Input: part model. Units: mm. Frame: model coordinates. A direction names the side the tool comes from. Round coordinates to 2 decimals unless told otherwise and drop trailing zeros. Loops run counter-clockwise (first coordinate to the right, second up) from the corner with the lowest first, then second, coordinate; pieces in that order, holes last.
1) Ray query, line 1 along X through (y, z) = (82, 29.5); line 2 along X through (y, z) = (100, 28); line 3 along Z through (x, y) = (10.5, 105.5). Return the intervals inside material, ascending.
2) Draft query along X for faces 3 (the face through (1.87, 75.13, 88.88)), 4 (the face through (0.1, 75.1, 76.2)), 5 (the face through (0, 152.4, 78)). Return one class per face: pulls with the +X half, pulls with the -X half, needs draft (parallel to the pull), parting line crosses it, or undercut.
3) Section B-B, the plane z = 65. Return loops of the section in (x, y), and give its area (3 significant figures).
4) Access query for faces 1 (the face through (0, 0, 78)), 2 (the face through (58.95, 75.13, 57.79)). Directions: +Z, -Z, +X, -X, +Y, -Y. A direction counts if a zero-diameter tool reaches every point of the face in a straight line with its end or side. Return the directions, or none.
5) First-contact query: pin 1 (1.5 mm diameter, centred on y = 99, z = 43, fed in from +X); pin 2 (0.6 mm diameter, centred on x = 82.5, y = 42.5, fed in from -Z); pin 3 (0.6 mm diameter, centred on x = -88.5, y = 108.5, fed in from -Z). Flat tips, straight axial feed; report the tip coordinate or a pass-through.
6) Section A-A, the plane y = 99.5. Return loops of the section in (x, z).
7) Section C-C, the plane z = 38. Return loops of the section in (x, y).
8) Section D-D, the plane x = -49.5. Return loops of the section in (y, z).
from build123d import *

# Parameters (mm, degrees)
F0_R     = 88.9
F1_DEPTH = 152.4
F4_DEPTH = 152.401
F5_DEPTH = 152.401
F7_DEPTH = 152.401


with BuildPart() as f1:
    # F0 (on Front) → F1 (new body)
    with BuildSketch(Plane.XZ):
        Circle(F0_R)
    extrude(amount=-F1_DEPTH)

    # F3 (on face) → F4 (cut, through all)
    with BuildSketch(Plane.XZ):
        with BuildLine():
            ThreePointArc((6.3453015162, 82.3057692308), (0, 76.2), (-6.3453015162, 82.3057692308))
            ThreePointArc((-6.3453015162, 82.3057692308), (-58.3716647869, 58.3716647869), (-82.3057692308, 6.3453015162))
            ThreePointArc((-82.3057692308, 6.3453015162), (-77.974338005, 4.4029328075), (-76.2, 0))
            ThreePointArc((-76.2, 0), (-77.974338005, -4.4029328075), (-82.3057692308, -6.3453015162))
            ThreePointArc((-82.3057692308, -6.3453015162), (-58.3716647869, -58.3716647869), (-6.3453015162, -82.3057692308))
            ThreePointArc((-6.3453015162, -82.3057692308), (0, -76.2), (6.3453015162, -82.3057692308))
            ThreePointArc((6.3453015162, -82.3057692308), (58.3716647869, -58.3716647869), (82.3057692308, -6.3453015162))
            ThreePointArc((82.3057692308, -6.3453015162), (76.2, 0), (82.3057692308, 6.3453015162))
            ThreePointArc((82.3057692308, 6.3453015162), (58.3716647869, 58.3716647869), (6.3453015162, 82.3057692308))
        make_face()
    extrude(amount=-F4_DEPTH, mode=Mode.SUBTRACT)

    # F2 (on face) → F5 (cut, through all)
    with BuildSketch(Plane.XZ):
        with BuildLine():
            ThreePointArc((-2.7935998838, 82.5027169231), (-1.9588679235, 80.5576966952), (0, 79.756))
            ThreePointArc((0, 79.756), (1.9588679235, 80.5576966952), (2.7935998838, 82.5027169231))
            ThreePointArc((2.7935998838, 82.5027169231), (2.7938999692, 82.5263576151), (2.794, 82.55))
            ThreePointArc((2.794, 82.55), (-0.0236423849, 85.3438999692), (-2.7935998838, 82.5027169231))
        make_face()
        with BuildLine():
            ThreePointArc((-82.5027169231, 2.7935998838), (-85.344, 0), (-82.5027169231, -2.7935998838))
            ThreePointArc((-82.5027169231, -2.7935998838), (-80.5576966952, -1.9588679235), (-79.756, 0))
            ThreePointArc((-79.756, 0), (-80.5576966952, 1.9588679235), (-82.5027169231, 2.7935998838))
        make_face()
        with BuildLine():
            ThreePointArc((79.756, 0), (80.5576966952, -1.9588679235), (82.5027169231, -2.7935998838))
            ThreePointArc((82.5027169231, -2.7935998838), (84.5088679235, -1.9923033048), (85.344, 0))
            ThreePointArc((85.344, 0), (84.5088679235, 1.9923033048), (82.5027169231, 2.7935998838))
            ThreePointArc((82.5027169231, 2.7935998838), (80.5576966952, 1.9588679235), (79.756, 0))
        make_face()
        with BuildLine():
            ThreePointArc((2.794, -82.55), (2.7938999692, -82.5263576151), (2.7935998838, -82.5027169231))
            ThreePointArc((2.7935998838, -82.5027169231), (1.9588679235, -80.5576966952), (0, -79.756))
            ThreePointArc((0, -79.756), (-1.9588679235, -80.5576966952), (-2.7935998838, -82.5027169231))
            ThreePointArc((-2.7935998838, -82.5027169231), (-0.0236423849, -85.3438999692), (2.794, -82.55))
        make_face()
    extrude(amount=-F5_DEPTH, mode=Mode.SUBTRACT)

    # F6 (on face) → F7 (cut, through all)
    with BuildSketch(Plane.XZ):
        with BuildLine():
            Line((82.55, 0), (76.2, 0))
            ThreePointArc((76.2, 0), (77.974338005, -4.4029328075), (82.3057692308, -6.3453015162))
            ThreePointArc((82.3057692308, -6.3453015162), (58.3716647869, -58.3716647869), (6.3453015162, -82.3057692308))
            ThreePointArc((6.3453015162, -82.3057692308), (0, -76.2), (-6.3453015162, -82.3057692308))
            ThreePointArc((-6.3453015162, -82.3057692308), (-58.3716647869, -58.3716647869), (-82.3057692308, -6.3453015162))
            ThreePointArc((-82.3057692308, -6.3453015162), (-77.974338005, -4.4029328075), (-76.2, 0))
            Line((-76.2, 0), (-88.9, 0))
            Line((-88.9, 0), (-104.8936669013, -139.8783236514))
            Line((-104.8936669013, -139.8783236514), (114.9751045783, -122.2419444763))
            Line((114.9751045783, -122.2419444763), (88.9, 0))
            Line((88.9, 0), (82.55, 0))
        make_face()
        Polygon((88.9, 6.35), (88.9, 0), (114.9751045783, -122.2419444763), (179.3332546949, -117.0795708895), (106.4055040479, 6.35), align=None)
        with BuildLine():
            ThreePointArc((82.3057692308, 6.3453015162), (77.974338005, 4.4029328075), (76.2, 0))
            Line((76.2, 0), (82.55, 0))
            Line((82.55, 0), (88.9, 0))
            Line((88.9, 0), (88.9, 6.35))
            Line((88.9, 6.35), (88.138, 6.35))
            ThreePointArc((88.138, 6.35), (85.598, 3.81), (83.058, 6.35))
            Line((83.058, 6.35), (82.55, 6.35))
            Line((82.55, 6.35), (82.3054068698, 6.35))
            ThreePointArc((82.3054068698, 6.35), (82.3055880838, 6.3476507607), (82.3057692308, 6.3453015162))
        make_face()
        with BuildLine():
            Line((-88.9, 0), (-76.2, 0))
            ThreePointArc((-76.2, 0), (-77.974338005, 4.4029328075), (-82.3057692308, 6.3453015162))
            ThreePointArc((-82.3057692308, 6.3453015162), (-82.3055880838, 6.3476507607), (-82.3054068698, 6.35))
            Line((-82.3054068698, 6.35), (-82.55, 6.35))
            Line((-82.55, 6.35), (-83.058, 6.35))
            ThreePointArc((-83.058, 6.35), (-85.598, 3.81), (-88.138, 6.35))
            Line((-88.138, 6.35), (-88.9, 6.35))
            Line((-88.9, 6.35), (-88.9, 0))
        make_face()
    extrude(amount=-F7_DEPTH, mode=Mode.SUBTRACT)


solid = f1.part
Final values:
1. line 1: x = -83.86 to -77.1, 77.1 to 83.86
1. line 2: x = -84.38 to -77.66, 77.66 to 84.38
1. line 3: z = 81.88 to 88.28
2. face 3: parting line crosses it
2. face 4: undercut
2. face 5: needs draft
3. outline: (-60.65, 0) - (-50.89, 0) - (-50.89, 152.4) - (-60.65, 152.4) - close; (50.89, 0) - (60.65, 0) - (60.65, 152.4) - (50.89, 152.4) - close
3. area: 2,980 mm2
4. face 1: +Z, -Z, +X, -X, -Y
4. face 2: -Z, +Y, -Y
5. pin 1: stops at x = 78.22
5. pin 2: stops at z = 6.35
5. pin 3: stops at z = 6.35
6. outline: (-88.67, 6.35) - (-88.14, 6.35) arc R2.54 ccw to (-83.06, 6.35) - (-82.31, 6.35) arc R82.55 cw to (-6.35, 82.31) arc R6.35 ccw to (6.35, 82.31) arc R82.55 cw to (82.31, 6.35) - (83.06, 6.35) arc R2.54 ccw to (88.14, 6.35) - (88.67, 6.35) arc R88.9 ccw to start; hole circle Ø5.59 at (0, 82.55)
7. outline: (-80.37, 0) - (-73.28, 0) - (-73.28, 152.4) - (-80.37, 152.4) - close; (73.28, 0) - (80.37, 0) - (80.37, 152.4) - (73.28, 152.4) - close
8. outline: (0, 66.06) - (152.4, 66.06) - (152.4, 73.84) - (0, 73.84) - close
